from build123d import *

# Parameters (mm, degrees)
SKETCH1_R           = 39
SKETCH1_R_2         = 4
SKETCH1_R_3         = 9.5
BOSS_EXTRUDE1_DEPTH = 18


with BuildPart() as part:
    # Sketch1 → Boss-Extrude1 (new body)
    with BuildSketch(Plane.XY):
        Circle(SKETCH1_R)
        with Locations((-21.213203436, 21.213203436)):
            Circle(SKETCH1_R_2, mode=Mode.SUBTRACT)
        with Locations((21.213203436, 21.213203436)):
            Circle(SKETCH1_R_2, mode=Mode.SUBTRACT)
        with Locations((21.213203436, -21.213203436)):
            Circle(SKETCH1_R_2, mode=Mode.SUBTRACT)
        with Locations((-21.213203436, -21.213203436)):
            Circle(SKETCH1_R_2, mode=Mode.SUBTRACT)
        Circle(SKETCH1_R_3, mode=Mode.SUBTRACT)
    extrude(amount=BOSS_EXTRUDE1_DEPTH)


solid = part.part
Can you work these out from the model? Positions are in its coordinate system, mm. Give positions to 0.01 mm unless a question says otherwise; leave off trailing zeros. Order: outer loops, then holes, each group sorted by start corner. A loop starts at its lowest first (then second) coordinate and runs counter-clockwise, first axis right, second up. Notation, with made-up numbers: M 50.25,5.25 L 69.25,5.25 A26 cw 69.25,21.25 Z; hole C -27,10 d9. An arc over 180 degrees is marked long. One line per question, with ' | ' between items.
Item 1: Suppose I cut it at A-A, the plane x = 0. Write out the boundary of the cut face in (y, z).
Answer block:
outline: M -39,0 L -9.5,0 L -9.5,18 L -39,18 Z; M 9.5,0 L 39,0 L 39,18 L 9.5,18 Z
Item 2: I'm going to push flat-ended pins straight in: pin 1 Ø2 at (x, z) = (10.5, 15.5) entering from -Y; pin 2 Ø2 at (y, z) = (-30.5, 14) entering from +X; pin 3 Ø10 at (x, z) = (-18.5, 9.5) entering from +Y; pin 4 Ø7 at (x, y) = (21.21, -21.21) entering from -Z. Where does each tip first touch, or does it pass through?
Answer block:
pin 1: stops at y = -37.83 | pin 2: stops at x = 25.51 | pin 3: stops at y = 36.59 | pin 4: passes through
Item 3: We'd pull the mould along Y, two halves only. Please class faces 1 (the face through (-24.16, -18.51, 8.87)), 2 (the face through (8, -8, 18)), 3 (the face through (-5.077, 38.668, 8.874)): released by +Y, released by -Y, zero draft, split by the parting line, or undercut.
Answer block:
face 1: undercut | face 2: zero draft | face 3: split by the parting line
Item 4: Suppose I cut it at D-D, the plane y = 23. Write out the boundary of the cut face in (x, z).
Answer block:
outline: M -31.5,0 L -24.79,0 L -24.79,18 L -31.5,18 Z; M -17.63,0 L 17.63,0 L 17.63,18 L -17.63,18 Z; M 24.79,0 L 31.5,0 L 31.5,18 L 24.79,18 Z
Item 5: Please list where these lines run through material, in increasing order: L1, parallel to X at y = 22, z = 12.5; L2, parallel to X at y = -19, z = 12.5; L3, parallel to X at y = -35, z = 6.75.
Answer block:
L1: x = -32.2 to -25.14, -17.29 to 17.29, 25.14 to 32.2 | L2: x = -34.06 to -24.55, -17.88 to 17.88, 24.55 to 34.06 | L3: x = -17.2 to 17.2
Item 6: Suppose I cut it at C-C, the plane z = 3. Write out the boundary of the cut face in (x, y), then the cut area to 3 significant figures.
Answer block:
outline: C 0,0 d78; hole C -21.21,-21.21 d8; hole C -21.21,21.21 d8; hole C 0,0 d19; hole C 21.21,-21.21 d8; hole C 21.21,21.21 d8 | area: 4,290 mm2
